Input: dimensioned drawing with shaded views. Units: mm. Origin: part minimum x, y, z. A direction names the side the tool comes from. Round coordinates to 2 decimals unless told otherwise and drop trailing zeros. Loops run counter-clockwise (first coordinate to the right, second up) from the corner with the lowest first, then second, coordinate; pieces in that order, holes last. Notation, with made-up numbers: (-35, 39.5) - (-6, 39.5) arc R25 cw to (-6, 74.5) - close; hole circle Ø1 at (28, 59.25). An arc over 180 degrees is marked (long way). Answer as a JSON object with one key per item and string values. Group by question number.
Item 1: Section D-D (z = 1.75). Return the cut outline in (x, y), plus the area to 3 significant figures.
Item 2: Section B-B (y = 13). Return the cut outline in (x, z).
Item 3: Line query: line 1 (X direction, y = 22.15, z = 4); line 2 (X direction, y = 1.4, z = 4); line 3 (X direction, y = 6.25, z = 4.5). Output: solid intervals per line, ascending.
Item 4: Draft query along X for the marked faces 4, 5, 6 and 7. Return one class per face: released by +X, released by -X, zero draft, split by the parting line, or undercut.
Item 5: Section C-C (z = 4.25). Return the cut outline in (x, y), plus the area to 3 significant figures.
Item 6: Section A-A (x = 19.75). Return the cut outline in (y, z).
Item 7: Reachability of the marked faces 1, 2 and 3 from +Z, -Z, +X, -X, +Y, -Y: full face, straight path, thin tool, end or side. Return the list, or none.
Item 8: First-contact query: pin 1 (2.5 mm diameter, centred on x = 4, z = 5, fed in from +Y); pin 2 (1.5 mm diameter, centred on x = 11, y = 19, fed in from -Z); pin 3 (2.5 mm diameter, centred on y = 8.5, z = 3.5, fed in from -X); pin 4 (2.5 mm diameter, centred on x = 4, z = 4, fed in from +Y). Flat tips, straight axial feed; report the tip coordinate or a pass-through.
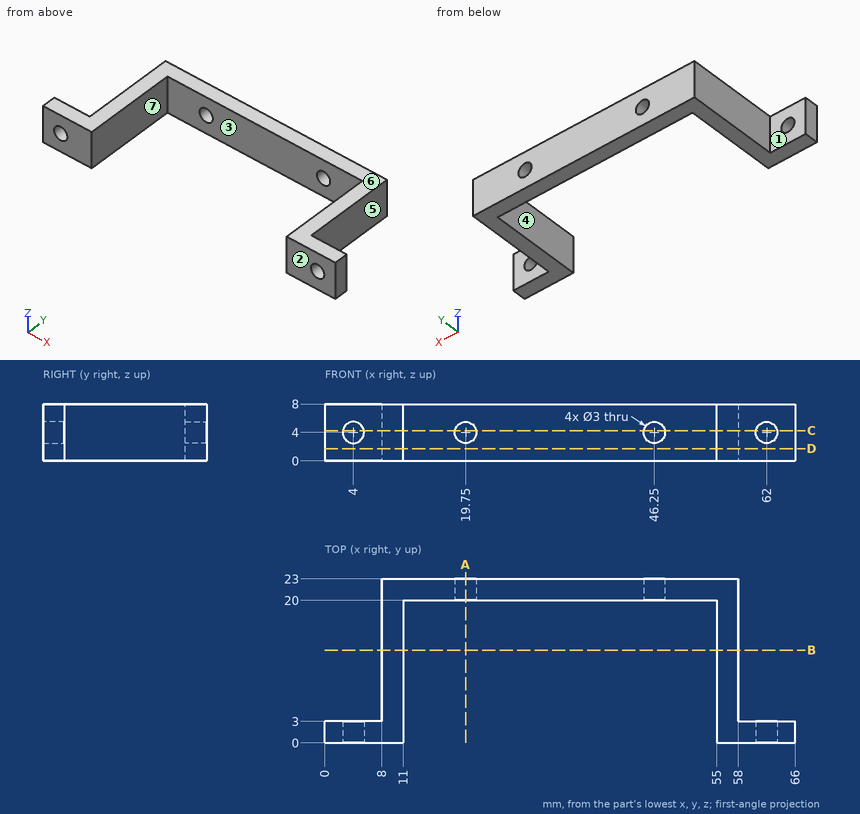
Values:
{
 "1": {"outline": "(0, 0) - (11, 0) - (11, 20) - (55, 20) - (55, 0) - (66, 0) - (66, 3) - (58, 3) - (58, 23) - (8, 23) - (8, 3) - (0, 3) - close", "area": "318 mm^2"},
 "2": {"outline": "(8, 0) - (11, 0) - (11, 8) - (8, 8) - close; (55, 0) - (58, 0) - (58, 8) - (55, 8) - close"},
 "3": {"line 1": "x = 8 to 18.25, 21.25 to 44.75, 47.75 to 58", "line 2": "x = 0 to 2.5, 5.5 to 11, 55 to 60.5, 63.5 to 66", "line 3": "x = 8 to 11, 55 to 58"},
 "4": {"face 4": "undercut", "face 5": "released by +X", "face 6": "zero draft", "face 7": "undercut"},
 "5": {"outline": "(0, 0) - (2.52, 0) - (2.52, 3) - (0, 3) - close; (5.48, 0) - (11, 0) - (11, 20) - (18.27, 20) - (18.27, 23) - (8, 23) - (8, 3) - (5.48, 3) - close; (21.23, 20) - (44.77, 20) - (44.77, 23) - (21.23, 23) - close; (47.73, 20) - (55, 20) - (55, 0) - (60.52, 0) - (60.52, 3) - (58, 3) - (58, 23) - (47.73, 23) - close; (63.48, 0) - (66, 0) - (66, 3) - (63.48, 3) - close", "area": "283 mm^2"},
 "6": {"outline": "(20, 0) - (23, 0) - (23, 2.5) - (20, 2.5) - close; (20, 5.5) - (23, 5.5) - (23, 8) - (20, 8) - close"},
 "7": {"face 1": "+Z, -Z, -X, +Y", "face 2": "+Z, -Z, +X, -X, -Y", "face 3": "+Z, -Z, -Y"},
 "8": {"pin 1": "stops at y = 3", "pin 2": "stops at z = 0", "pin 3": "stops at x = 8", "pin 4": "passes through"}
}
